Can you work these out from the model? Positions are in its coordinate system, mm. A direction names the side the tool comes from. Round coordinates to 2 decimals unless told otherwise and drop trailing zeros. Order: outer loops, then holes, each group sorted by start corner. A loop starts at its lowest first (then second) coordinate and runs counter-clockwise, first axis right, second up. Notation, with made-up numbers: (79.5, 11) - (126.5, 11) arc R22 ccw to (126.5, 33) - close; hole circle Ø8 at (53.5, 5.5). An arc over 180 degrees is marked (long way). Write item = value, one per line.
from build123d import *

# Parameters (mm, degrees)
SKETCH1_R           = 31.25
SKETCH1_R_2         = 3
BOSS_EXTRUDE1_DEPTH = 8
SKETCH2_R           = 33.75
SKETCH2_R_2         = 3
BOSS_EXTRUDE2_DEPTH = 1


with BuildPart() as part:
    # Sketch1 → Boss-Extrude1 (new, symmetric)
    with BuildSketch(Plane.XY):
        Circle(SKETCH1_R)
        Circle(SKETCH1_R_2, mode=Mode.SUBTRACT)
    extrude(amount=BOSS_EXTRUDE1_DEPTH, both=True)

    # Sketch2 → Boss-Extrude2 (add, symmetric)
    with BuildSketch(Plane.XY.offset(8)):
        Circle(SKETCH2_R)
        Circle(SKETCH2_R_2, mode=Mode.SUBTRACT)
    boss_extrude2 = extrude(amount=BOSS_EXTRUDE2_DEPTH, both=True)

    # Mirror1: Boss-Extrude2 across plane
    add(boss_extrude2.mirror(Plane.XY))


solid = part.part
(1) On a 3-axis mill with a long thin cutter (end or side, diameter ignored), from which of +Z, -Z, +X, -X, +Y, -Y can I reach the whole of each face in a straight line? I mean faces 1 (the face through (0, -7, -9)), 2 (the face through (10, -30, -7)). Say none if no direction works.
Computed:
face_1 = -Z, +X, -X, +Y, -Y
face_2 = none
(2) If we section it at C-C (z = 2.75): Write out the boundary of the cut face in (x, y).
Computed:
outline = circle Ø62.5 at (0, 0); hole circle Ø6 at (0, 0)
(3) Will these pins go through, and if not, where does the flat tip stop? P1, Ø1, axis at y = -14.5, z = -4.5, coming from the +X side; P2, Ø1.5, axis at x = -1.5, z = 1, coming from the -Y side; P3, Ø4, axis at x = 5, z = 2.5, coming from the +Y side; P4, Ø8, axis at x = 0, y = 0, coming from the +Z side.
Computed:
P1 = 27.94
P2 = -31.24
P3 = 31.11
P4 = 9
(4) If we section it at D-D (y = 28.5): Write out the boundary of the cut face in (x, z).
Computed:
outline = (-18.08, -9) - (18.08, -9) - (18.08, -7) - (12.82, -7) - (12.82, 7) - (18.08, 7) - (18.08, 9) - (-18.08, 9) - (-18.08, 7) - (-12.82, 7) - (-12.82, -7) - (-18.08, -7) - close
(5) Thinking about a two-plate mould opening in Z: for faces 3 (the face through (-26.78, -20.54, -8.01)), 4 (the face through (10, -30, 7)), 5 (the face through (0, -7, 9)), 6 (the face through (-31.22, 1.37, 0.1)), which applies, +Z half, -Z half, draft (parallel to the pull), parting line (faces both ways), or undercut?
Computed:
face_3 = draft
face_4 = undercut
face_5 = +Z half
face_6 = undercut
(6) If we section it at A-A (y = 0): Write out the boundary of the cut face in (x, z).
Computed:
outline = (-33.75, -9) - (-3, -9) - (-3, 9) - (-33.75, 9) - (-33.75, 7) - (-31.25, 7) - (-31.25, -7) - (-33.75, -7) - close; (3, -9) - (33.75, -9) - (33.75, -7) - (31.25, -7) - (31.25, 7) - (33.75, 7) - (33.75, 9) - (3, 9) - close
(7) If I drill on line 1 (Y direction, x = 0, z = -7.75); line 2 (X direction, y = 0.5, z = 2); line 3 (Y direction, x = 2, z = 1), over which ranges is the centre line in solid material (lowest first)? Write a range as from..to.
Computed:
line_1 = -33.75..-3, 3..33.75
line_2 = -31.25..-2.96, 2.96..31.25
line_3 = -31.19..-2.24, 2.24..31.19
